Input: part model. Units: mm. Frame: model coordinates. Coordinates: 2 decimals unless noted, no trailing zeros. Order: outer loops, then holes, each group sorted by start corner. A loop starts at its lowest first (then second) coordinate and runs counter-clockwise, first axis right, second up. Notation, with made-up numbers: (59, 10) -> (118, 10) arc R19 cw to (118, 18) -> close; hole circle Ø2 at (47, -37). An arc over 180 degrees is marked (long way). Use one line per item in the form item = value. Start each with the question number.
1) Section query C-C on x = 8.5. Output: boundary loops of the cut face in (y, z).
2) Pin query (flat end, axial travel): pin 1 (5 mm diameter, centred on x = 6.5, y = -0.5, fed in from -Z); pin 2 (2 mm diameter, centred on x = 3, z = -6, fed in from -Y); pin 3 (1.5 mm diameter, centred on x = 3, z = -6.5, fed in from +Y); pin 4 (13.5 mm diameter, centred on y = 0, z = 0, fed in from -X). Return the tip coordinate at first contact, or that it passes through.
3) Section query A-A on x = 4.5. Output: boundary loops of the cut face in (y, z), then the cut area to 3 significant figures.
4) Draft query along Y for faces 1 (the flat face through (10, 6, -6)), 2 (the cylindrical face through (4.93, -7.493, -0.33)), 3 (the flat face through (5.07, 11.299, -6.507)). Return one class per face: pulls with the +Y half, pulls with the -Y half, needs draft (parallel to the pull), parting line crosses it, or undercut.
5) Ray query, line 1 along Y through (x, z) = (6.75, 6); line 2 along Z through (x, y) = (3.5, 0); line 3 along Z through (x, y) = (5, 5.5). Return the intervals inside material, ascending.
Autodesk Inventor part; units mm, degrees
ref_plane "YZ Plane" through (0, 0, 0) normal (1, 0, 0) x (0, 1, 0)
ref_plane "XZ Plane" through (0, 0, 0) normal (0, 1, 0) x (-1, 0, 0)
ref_plane "XY Plane" through (0, 0, 0) normal (0, 0, 1) x (1, 0, 0)
sketch "Sketch4" plane through (0, 0, 0) normal (1, 0, 0) x (0, 1, 0)
  circle A0 centre (0, 0) radius 7.5
  circle A1 centre (0, 0) radius 15
  dimension "d12" = 15
  dimension "d13" = 30
extrude "Extrusion3" add sketch "Sketch4" along normal blind 10
fillet "Fillet1" radius 2 2 edges at (10, -15, 0) (0, -15, 0)
sketch "Sketch6" plane through (10, 0, 0) normal (1, 0, 0) x (0, 0, -1)
  line L0 (-12.986, 7.6174) -> (0.1038, 15.0549)
  line L1 (0.1038, 15.0549) -> (13.0898, 7.4376)
  line L2 (13.0898, 7.4376) -> (12.986, -7.6174)
  line L3 (12.986, -7.6174) -> (-0.1038, -15.0549)
  line L4 (-0.1038, -15.0549) -> (-13.0898, -7.4376)
  line L5 (-13.0898, -7.4376) -> (-12.986, 7.6174)
  circle A0 centre (0, 0) radius 17.8514
  circle A1 centre (0, 0) radius 7.5945
extrude "Extrusion4" cut sketch "Sketch6" against normal blind 10 contours A0
properties part number "Nut" material "Steel, Carbon"
Answers below:
q1.outline = (-14.94, -0.11) -> (-7.74, -12.78) arc R14.94 ccw to (-7.38, -12.99) -> (7.2, -13.09) arc R14.94 ccw to (7.56, -12.88) -> (14.93, -0.31) arc R14.94 ccw to (14.94, 0.11) -> (7.74, 12.78) arc R14.94 ccw to (7.38, 12.99) -> (-7.2, 13.09) arc R14.94 ccw to (-7.56, 12.88) -> (-14.93, 0.31) arc R14.94 ccw to start; hole circle Ø15 at (0, 0)
q2.pin_1 = -13.05
q2.pin_2 = -12.15
q2.pin_3 = 11.74
q2.pin_4 = through
q3.outline = (-15, 0.01) -> (-7.67, -12.89) arc R15 ccw to (-7.51, -12.99) -> (7.33, -13.09) arc R15 ccw to (7.49, -12.99) -> (15, -0.2) arc R15 ccw to (15, -0.01) -> (7.67, 12.89) arc R15 ccw to (7.51, 12.99) -> (-7.33, 13.09) arc R15 ccw to (-7.49, 12.99) -> (-15, 0.2) arc R15 ccw to start; hole circle Ø15 at (0, 0)
q3.area = 412 mm^2
q4.face_1 = needs draft
q4.face_2 = undercut
q4.face_3 = pulls with the +Y half
q5.line_1 = -11.6 to -4.5, 4.5 to 11.59
q5.line_2 = -13.04 to -7.5, 7.5 to 13.04
q5.line_3 = -13.08 to -5.1, 5.1 to 13
